from build123d import *

# Parameters (mm, degrees)
SKETCH4_R           = 3.16
BOSS_EXTRUDE1_DEPTH = 30.5
CUT_EXTRUDE2_START  = -29
CUT_EXTRUDE2_DEPTH  = 29
SKETCH6_R           = 2.375
CUT_EXTRUDE3_DEPTH  = 5


with BuildPart() as part:
    # Sketch1 → Revolve1 (revolve)
    with BuildSketch(Plane(origin=(0, 0, 0), x_dir=(1, 0, 0), z_dir=(0, 1, 0))):
        Polygon((0, 0), (20.05, 0), (20.05, 53.2), (25.3, 53.2), (25.3, 88), (14.25, 88), (14.25, 89.5), (0, 89.5), align=None)
    revolve(axis=Axis((0, 0, 0), (0, 0, -1)))

    # Sketch4 → Boss-Extrude1 (add)
    with BuildSketch(Plane(origin=(0, 0, -89.5), x_dir=(-1, 0, 0), z_dir=(0, 0, -1))):
        with Locations(Location((0, 8.21, 0), (0, 0, 180))):
            Circle(SKETCH4_R)
    extrude(amount=BOSS_EXTRUDE1_DEPTH)

    # Sketch5 → Cut-Extrude2 (cut)
    with BuildSketch(Plane(origin=(0, 0, -120), x_dir=(-1, 0, 0), z_dir=(0, 0, -1)).offset(CUT_EXTRUDE2_START)):
        with BuildLine():
            Line((-2.370126579, 10.3), (2.370126579, 10.3))
            ThreePointArc((2.370126579, 10.3), (0, 11.37), (-2.370126579, 10.3))
        make_face()
    extrude(amount=CUT_EXTRUDE2_DEPTH, mode=Mode.SUBTRACT)

    # Sketch6 → Cut-Extrude3 (cut)
    with BuildSketch(Plane(origin=(0, 0, -88), x_dir=(-1, 0, 0), z_dir=(0, 0, -1))):
        with Locations((-19, 0)):
            Circle(SKETCH6_R)
        with Locations((19, 0)):
            Circle(SKETCH6_R)
    extrude(amount=-CUT_EXTRUDE3_DEPTH, mode=Mode.SUBTRACT)


solid = part.part
Model file for the job. Use its own axes, mm. A direction names the side the tool comes from. Give positions to 0.01 mm unless a question says otherwise; leave off trailing zeros. Loops run counter-clockwise (first coordinate to the right, second up) from the corner with the lowest first, then second, coordinate; pieces in that order, holes last.
1) Saw through at D-D (y = -7). Write the cut outline in (x, z), plus the area to 3 significant figures.
2) Saw through at C-C (z = -96.5). Write the cut outline in (x, y), plus the area to 3 significant figures.
3) Flat gauge pins, fed straight in: pin 1 Ø12 at (x, y) = (-12.5, 6.5) entering from -Z; pin 2 Ø2 at (x, y) = (-19.5, 4) entering from -Z; pin 3 Ø8 at (x, z) = (18.5, -43.5) entering from +Y; pin 4 Ø15 at (x, y) = (-3, -3) entering from +Z. Where does each tip first touch, or does it go through?
4) Tool access for faces 4 (the flat face through (8, -19, -53.2)), 5 (the flat face through (-19, 0, -83)), 6 (the flat face through (0, 8, -120)), 7 (the flat face through (0, 10.3, -105)): list every direction of +Z, -Z, +X, -X, +Y, -Y with a clear straight run to the whole face (end or side of a thin tool).
5) Saw through at B-B (x = 0). Write the cut outline in (y, z).
6) Saw through at A-A (y = 0). Write the cut outline in (x, z) (3 decimals), plus the area to 3 significant figures.
7) Wall check: line 1 (Z direction, x = -20.5, y = 13); line 2 (Z direction, x = 5.5, y = -16.5); line 3 (Y direction, x = 19, z = -86.15) (3 decimals). Give the ranges that are in metal, low to high.
8) Pull direction Y, two halves, no side cores. Call faces 1 (the cylindrical face through (-5.48, 24.7, -70.84)), 2 (the flat face through (0, 0, 0)), 3 (the cylindrical face through (16.735, 0.713, -85.535)): +Y half, -Y half, draft (parallel to the pull), parting line (faces both ways), or undercut.
Answer block:
1. outline: (-24.31, -88) - (-12.41, -88) - (-12.41, -89.5) - (12.41, -89.5) - (12.41, -88) - (24.31, -88) - (24.31, -53.2) - (18.79, -53.2) - (18.79, 0) - (-18.79, 0) - (-18.79, -53.2) - (-24.31, -53.2) - close
1. area: 3,730 mm2
2. outline: (-2.37, 10.3) arc R3.16 ccw (long way) to (2.37, 10.3) - close
2. area: 27.9 mm2
3. pin 1: stops at z = -89.5
3. pin 2: stops at z = -88
3. pin 3: stops at y = 13.85
3. pin 4: stops at z = 0
4. face 4: +Z
4. face 5: -Z
4. face 6: -Z, +X, -X, +Y, -Y
4. face 7: -Z, +X, -X, +Y
5. outline: (-25.3, -88) - (-14.25, -88) - (-14.25, -89.5) - (5.05, -89.5) - (5.05, -120) - (10.3, -120) - (10.3, -91) - (11.37, -91) - (11.37, -89.5) - (14.25, -89.5) - (14.25, -88) - (25.3, -88) - (25.3, -53.2) - (20.05, -53.2) - (20.05, 0) - (-20.05, 0) - (-20.05, -53.2) - (-25.3, -53.2) - close
6. outline: (-25.3, -88) - (-21.375, -88) - (-21.375, -83) - (-16.625, -83) - (-16.625, -88) - (-14.25, -88) - (-14.25, -89.5) - (14.25, -89.5) - (14.25, -88) - (16.625, -88) - (16.625, -83) - (21.375, -83) - (21.375, -88) - (25.3, -88) - (25.3, -53.2) - (20.05, -53.2) - (20.05, 0) - (-20.05, 0) - (-20.05, -53.2) - (-25.3, -53.2) - close
6. area: 3,890 mm2
7. line 1: z = -88 to -53.2
7. line 2: z = -88 to 0
7. line 3: y = -16.706 to -2.375, 2.375 to 16.706
8. face 1: parting line
8. face 2: draft
8. face 3: undercut
